```python
from build123d import *

# Parameters (mm, degrees)
EXTRUDE_1_DEPTH     = 19
SKETCH_3_W          = 23.2
SKETCH_3_H          = 9
CUT_EXTRUDE_2_DEPTH = 31.8
CUT_EXTRUDE_3_DEPTH = 8
SKETCH_5_W          = 7.5
SKETCH_5_H          = 7.5
CUT_EXTRUDE_4_DEPTH = 31.8
SKETCH_7_R          = 0.75
CUT_EXTRUDE_6_DEPTH = 31.8
FILLET_3_R          = 2
FILLET_4_R          = 0.5
SKETCH_8_R          = 0.95
EXTRUDE_2_DEPTH     = 5


with BuildPart() as part:
    # 草图1 → 凸台-拉伸1 (new body)
    with BuildSketch(Plane(origin=(0, 0, 0), x_dir=(1, 0, 0), z_dir=(0, 1, 0))):
        Polygon((-5.22, 18.4025), (-2.42, 18.4025), (-2.42, -6.5975), (20.78, -6.5975), (20.78, -12.3975), (-5.22, -12.3975), align=None)
    extrude(amount=EXTRUDE_1_DEPTH)

    # 草图3 → 切除-拉伸2 (cut, through all)
    with BuildSketch(Plane.XY.offset(12.3975)):
        with Locations((9.18, 14.5)):
            Rectangle(SKETCH_3_W, SKETCH_3_H)
    extrude(amount=-CUT_EXTRUDE_2_DEPTH, mode=Mode.SUBTRACT)

    # 草图4 → 切除-拉伸3 (cut)
    with BuildSketch(Plane(origin=(0, 10, 0), x_dir=(1, 0, 0), z_dir=(0, 1, 0))):
        with BuildLine():
            Line((-0.82, -8.4975), (19.18, -8.4975))
            ThreePointArc((19.18, -8.4975), (20.18, -9.4975), (19.18, -10.4975))
            Line((19.18, -10.4975), (-0.82, -10.4975))
            ThreePointArc((-0.82, -10.4975), (-1.82, -9.4975), (-0.82, -8.4975))
        make_face()
    extrude(amount=-CUT_EXTRUDE_3_DEPTH, mode=Mode.SUBTRACT)

    # 草图5 → 切除-拉伸4 (cut, through all)
    with BuildSketch(Plane.XY.offset(12.3975)):
        with Locations((9.18, 6.25)):
            Rectangle(SKETCH_5_W, SKETCH_5_H)
    extrude(amount=-CUT_EXTRUDE_4_DEPTH, mode=Mode.SUBTRACT)

    # 草图7 → 切除-拉伸6 (cut, through all)
    with BuildSketch(Plane.XY.offset(12.3975)):
        with Locations((2.88, 6.2)):
            Circle(SKETCH_7_R)
        with Locations((15.48, 6.2)):
            Circle(SKETCH_7_R)
    extrude(amount=-CUT_EXTRUDE_6_DEPTH, mode=Mode.SUBTRACT)

    # 圆角3
    fillet_3_edges = [part.edges().sort_by_distance(p)[0] for p in [
        (20.78, 5, 6.5975),
        (20.78, 5, 12.3975),
    ]]
    fillet(fillet_3_edges, radius=FILLET_3_R)

    # 圆角4
    fillet_4_edges = [part.edges().sort_by_distance(p)[0] for p in [
        (-2.42, 14.5, 12.3975),
    ]]
    fillet(fillet_4_edges, radius=FILLET_4_R)

    # 草图8 → 凸台-拉伸2 (add)
    with BuildSketch(Plane(origin=(-2.42, 0, 0), x_dir=(0, 0, -1), z_dir=(1, 0, 0))):
        with Locations((16.4025, 17)):
            Circle(SKETCH_8_R)
        with Locations((16.4025, 3.5)):
            Circle(SKETCH_8_R)
        with Locations((-4.5975, 3.5)):
            Circle(SKETCH_8_R)
        with Locations((-4.5975, 17)):
            Circle(SKETCH_8_R)
    extrude(amount=EXTRUDE_2_DEPTH)


solid = part.part
```
Model file for the job. Use its own axes, mm. A direction names the side the tool comes from. Coordinates: 2 decimals unless noted, no trailing zeros. Loops run counter-clockwise (first coordinate to the right, second up) from the corner with the lowest first, then second, coordinate; pieces in that order, holes last. Notation, with made-up numbers: (63, 51.25) - (122, 51.25) arc R26 ccw to (122, 85.25) - close; hole circle Ø9 at (-0.75, 86). An arc over 180 degrees is marked (long way). Write item = value, one per line. Start each with the question number.
Item 1: Pull direction Y, two halves, no side cores. Call faces 4 (the face through (5, 6, 8.498)), 5 (the face through (0.04, 4.14, -15.7)), 6 (the face through (1, 10, 11)): +Y half, -Y half, draft (parallel to the pull), parting line (faces both ways), or undercut.
Item 2: Saw through at B-B, the plane x = 15.48. List the corners of the cut face in (y, z), then the cut area to 3 significant figures.
Item 3: 3-axis set-ups, long thin cutter, end or side, ignore diameter. For faces 1 (the face through (0.045, 16.157, 4.159)), 2 (the face through (20.18, 6.06, 9.48)), 3 (the face through (5.43, 6, 8)): which of +Z, -Z, +X, -X, +Y, -Y reach the whole face in a straight line?
Item 4: Saw through at D-D, the plane y = 6.2. State how many separate pieces and enclosed holes the cut face has, then the cut area to 3 significant figures.
Item 5: Saw through at C-C, the plane x = 4.75. List the corners of the cut face in (y, z).
Item 6: Wall check: probe 1 along Y at (x, z) = (15.48, 7.9); probe 2 along Z at (x, y) = (2.5, 8); probe 3 along X at (y, z) = (5, 4.5). Give the ranges that are in metal, low to high. Write a range as [from, to].
Item 7: Saw through at A-A, the plane y = 9.25. List the corners of the cut face in (x, z), then the cut area to 3 significant figures.
Item 8: Drop flat-ended pins along their axis: pin 1 Ø1.4 at (x, y) = (2.88, 6.2) entering from -Z; pin 2 Ø3 at (x, z) = (15.5, 9) entering from +Y; pin 3 Ø2.5 at (x, y) = (15.48, 6.2) entering from -Z; pin 4 Ø0.6 at (x, z) = (7.5, 9.5) entering from +Y. Give the stop position or say it passes through.
Answers:
q1.face_4 = draft
q1.face_5 = undercut
q1.face_6 = +Y half
q2.outline = (0, 6.6) - (5.45, 6.6) - (5.45, 8.5) - (2, 8.5) - (2, 10.5) - (5.45, 10.5) - (5.45, 12.4) - (0, 12.4) - close; (6.95, 6.6) - (10, 6.6) - (10, 8.5) - (6.95, 8.5) - close; (6.95, 10.5) - (10, 10.5) - (10, 12.4) - (6.95, 12.4) - close
q2.area = 36.3 mm2
q3.face_1 = +X
q3.face_2 = +Y
q3.face_3 = +Z, -Z, +Y
q4.separate_pieces = 6
q4.enclosed_holes = 0
q4.area = 136 mm2
q5.outline = (0, 6.6) - (10, 6.6) - (10, 8.5) - (2, 8.5) - (2, 10.5) - (10, 10.5) - (10, 12.4) - (0, 12.4) - close
q6.probe_1 = [0, 5.45], [6.95, 10]
q6.probe_2 = [6.6, 8.5], [10.5, 12.4]
q6.probe_3 = [-5.22, -2.42]
q7.outline = (-5.22, -18.4) - (-2.42, -18.4) - (-2.42, 6.6) - (5.43, 6.6) - (5.43, 8.5) - (-0.82, 8.5) arc R1 cw to (-0.82, 10.5) - (5.43, 10.5) - (5.43, 12.4) - (-5.22, 12.4) - close; (12.93, 6.6) - (18.78, 6.6) arc R2 ccw to (20.78, 8.6) - (20.78, 10.4) arc R2 ccw to (18.78, 12.4) - (12.93, 12.4) - (12.93, 10.5) - (19.18, 10.5) arc R1 cw to (19.18, 8.5) - (12.93, 8.5) - close
q7.area = 147 mm2
q8.pin_1 = through
q8.pin_2 = 10
q8.pin_3 = 6.6
q8.pin_4 = 2
